from build123d import *

# Parameters (mm, degrees)
F0_W     = 100
F0_H     = 95
F0_R     = 3
F1_DEPTH = 6


with BuildPart() as f1:
    # F0 (on Front) → F1 (new body, symmetric)
    with BuildSketch(Plane.XZ):
        with Locations((42.5, 40)):
            Rectangle(F0_W, F0_H)
        Circle(F0_R, mode=Mode.SUBTRACT)
        with BuildLine():
            ThreePointArc((5.6215454072, 64.2545580269), (2.8944285412, 67.5046093494), (6.1444798637, 70.2317262155))
            ThreePointArc((6.1444798637, 70.2317262155), (49.8510280737, 49.8510280737), (70.2317262155, 6.1444798637))
            ThreePointArc((70.2317262155, 6.1444798637), (67.5046093494, 2.8944285412), (64.2545580269, 5.6215454072))
            ThreePointArc((64.2545580269, 5.6215454072), (45.6083873865, 45.6083873865), (5.6215454072, 64.2545580269))
        make_face(mode=Mode.SUBTRACT)
    extrude(amount=F1_DEPTH, both=True)


solid = f1.part
Geometry: final body of the model. Coordinates: model frame, mm. A direction names the side the tool comes from. Give positions to 0.01 mm unless a question says otherwise; leave off trailing zeros. Loops run counter-clockwise (first coordinate to the right, second up) from the corner with the lowest first, then second, coordinate; pieces in that order, holes last. Notation, with made-up numbers: (-14.5, 44) -> (34.5, 44) arc R14 cw to (34.5, 52) -> close; hole circle Ø1 at (81, 69). An arc over 180 degrees is marked (long way). Put each result on its own line as item: value.
1. Cut plane C-C (z = 35). Return the cut outline in (x, y).
Taken from the geometry:
outline: (-7.5, -6) -> (54.18, -6) -> (54.18, 6) -> (-7.5, 6) -> close; (61.2, -6) -> (92.5, -6) -> (92.5, 6) -> (61.2, 6) -> close
2. Cut plane B-B (y = 3.5). Return the cut outline in (x, z), plus the area to 3 significant figures.
Taken from the geometry:
outline: (-7.5, -7.5) -> (92.5, -7.5) -> (92.5, 87.5) -> (-7.5, 87.5) -> close; hole circle Ø6 at (0, 0); hole (5.62, 64.25) arc R64.5 cw to (64.25, 5.62) arc R3 ccw to (70.23, 6.14) arc R70.5 ccw to (6.14, 70.23) arc R3 ccw to start
area: 8,880 mm2
3. Set-up query: faces 4 (the cylindrical face through (49.4, -0.1, 50.3)), 5 (the flat face through (42, 0, -7.5)). Return all of +Z, -Z, +X, -X, +Y, -Y with unobstructed straight access to the full face (end or side cutting, diameter ignored); none if empty.
Taken from the geometry:
face 4: +Y, -Y
face 5: -Z, +X, -X, +Y, -Y
4. Cut plane A-A (x = 0). Return the cut outline in (y, z), plus the area to 3 significant figures.
Taken from the geometry:
outline: (-6, -7.5) -> (6, -7.5) -> (6, -3) -> (-6, -3) -> close; (-6, 3) -> (6, 3) -> (6, 87.5) -> (-6, 87.5) -> close
area: 1,070 mm2
5. Pull-direction query (Z, two-part tool) for faces 1 (the flat face through (42, 0, 87.5)), 2 (the flat face through (-7.5, 0, 39)), 3 (the cylindrical face through (46.05, -0.08, 45.16)); classes: released by +Z, released by -Z, zero draft, split by the parting line, or undercut.
Taken from the geometry:
face 1: released by +Z
face 2: zero draft
face 3: undercut
6. Ray query, line 1 along Z through (x, y) = (0, 2.25); line 2 along X through (y, z) = (1, 56); line 3 along Z through (x, y) = (41, -0.5). Return the intervals inside material, ascending. Write a range as [from, to].
Taken from the geometry:
line 1: z = [-7.5, -3], [3, 87.5]
line 2: x = [-7.5, 32], [42.83, 92.5]
line 3: z = [-7.5, 49.79], [57.35, 87.5]
